Autodesk Fusion 360 part; units mm, degrees
sketch "Sketch1" plane through (0, 0, 0) normal (0, 0, 1) x (1, 0, 0)
sketch "Sketch2" plane through (0, 0, 0) normal (0, 0, 1) x (1, 0, 0)
  line L0 (-5, -5) -> (95, -5)
  line L1 (95, -5) -> (95, 13)
  line L2 (95, 13) -> (-5, 13)
  line L3 (-5, 13) -> (-5, -5)
  line L4 (-5, 13) -> (11, 13)
  line L5 (95, 13) -> (79, 13)
  line L6 (11, 13) -> (79, 13)
  line L7 (79, 13) -> (79, 19)
  line L8 (79, 19) -> (11, 19)
  line L9 (11, 19) -> (11, 13)
  line L10 (11, -5) -> (79, -5)
  line L11 (79, -5) -> (79, -11)
  line L12 (79, -11) -> (11, -11)
  line L13 (11, -11) -> (11, -5)
  line L14 (11, -11) -> (-5, -5)
  line L15 (-5, 13) -> (11, 19)
  line L16 (79, 19) -> (95, 13)
  line L17 (95, -5) -> (79, -11)
  dimension "d1" = 100
  dimension "d2" = 18
  dimension "d3" = 16
  dimension "d4" = 16
  dimension "d5" = 68
  dimension "d6" = 6
  dimension "d7" = 68
  dimension "d8" = 6
extrude "Extrude1" add sketch "Sketch2" along normal blind 20
sketch "Sketch3" plane through (95, 0, 0) normal (1, 0, 0) x (0, 1, 0)
  line L0 (-5, 0) -> (13, 0)
  line L1 (13, 0) -> (13, 20)
  line L2 (13, 20) -> (-5, 20)
  line L3 (-5, 20) -> (-5, 0)
  line L4 (-5, 20) -> (4, 20)
  arc A0 (-5, 20) -> (13, 20) centre (4, 20) ccw
  dimension "d11" = 9
  dimension "d12" = 18
extrude "Extrude2" cut sketch "Sketch3" against normal blind 100 contours L2 L4 A0
sketch "Sketch4" plane through (0, 0, 0) normal (0, 0, 1) x (1, 0, 0)
  line L0 (79, -11) -> (69.5, -11)
  line L1 (69.5, -11) -> (69.5, 19)
  line L2 (69.5, 19) -> (79, 19)
  line L3 (79, 19) -> (79, -11)
  line L4 (11, -11) -> (20.5, -11)
  line L5 (20.5, -11) -> (20.5, 19)
  line L6 (20.5, 19) -> (11, 19)
  line L7 (11, 19) -> (11, -11)
  line L8 (20.5, -11) -> (32.5, -11)
  line L9 (32.5, -11) -> (32.5, 19)
  line L10 (32.5, 19) -> (20.5, 19)
  line L11 (20.5, 19) -> (20.5, -11)
  line L12 (69.5, -11) -> (57.5, -11)
  line L13 (57.5, -11) -> (57.5, 19)
  line L14 (57.5, 19) -> (69.5, 19)
  line L15 (69.5, 19) -> (69.5, -11)
  dimension "d15" = 9.5
  dimension "d16" = 30
  dimension "d17" = 9.5
  dimension "d18" = 30
  dimension "d19" = 12
  dimension "d20" = 30
  dimension "d21" = 12
  dimension "d22" = 30
extrude "Extrude3" add sketch "Sketch4" against normal blind 25 contours L1 L12 L13 L14 L15 | L5 L8 L9 L10 L11
sketch "Sketch5" plane through (13.3562, -35.6164, 0) normal (0.3511, -0.9363, 0) x (0.9363, 0.3511, 0)
  line L0 (70.1076, 0) -> (87.1957, 0)
  line L1 (87.1957, 0) -> (87.1957, 20)
  line L2 (87.1957, 20) -> (70.1076, 20)
  line L3 (70.1076, 20) -> (70.1076, 0)
sketch "Sketch6" plane through (0, 0, 0) normal (0, 0, 1) x (1, 0, 0)
  line L0 (-5, -5) -> (95, -5)
  line L1 (95, -5) -> (95, -11)
  line L2 (95, -11) -> (-5, -11)
  line L3 (-5, -11) -> (-5, -5)
extrude "Extrude4" add sketch "Sketch6" along normal blind 20
Geometry check sheet. Reference: the model listing, model coordinates, mm. A direction names the side the tool comes from. Round coordinates to 2 decimals unless told otherwise and drop trailing zeros. Loops run counter-clockwise (first coordinate to the right, second up) from the corner with the lowest first, then second, coordinate; pieces in that order, holes last. Notation, with made-up numbers: (58, -35) - (75, -35) arc R28 ccw to (75, -11) - close; hole circle Ø5 at (-20.75, 60). An arc over 180 degrees is marked (long way). Write each question's results on one line, items separated by ' | '. Start each with the question number.
Q1. Access from +Z, -Z, +X, -X, +Y, -Y to the whole of each face (thin tool, end or side, straight path). Record for faces 1 (the flat face through (8, 4, 0)), 2 (the flat face through (32.5, 4, -12)), 3 (the flat face through (69.5, 4, -12)).
Q2. Cross-section at C-C on y = 4. Enter the section's corners in (x, z), and give its area (3 significant figures).
Q3. Gauge pin test, flat ends, axial feed: P1, Ø7.5, axis at y = 10.5, z = -14, coming from the +X side; P2, Ø7.5, axis at y = 10.5, z = -12, coming from the -X side; P3, Ø7.5, axis at x = 83, y = 3, coming from the -Z side. Record the tip position at first contact, or that the pin passes through.
Q4. Cross-section at D-D on z = 16. Enter the section's corners in (x, y).
Q5. Cross-section at A-A on z = -5. Enter the section's corners in (x, y).
Q6. Cross-section at B-B on x = 18. Enter the section's corners in (y, z).
Q7. Release check for a two-part mould opening along Y. For faces 4 (the cylindrical face through (46, 4, 11)), 5 (the flat face through (46, -11, 7)), 6 (the flat face through (-5, 1, 8)) record: +Y half, -Y half, draft (parallel to the pull), parting line (faces both ways), or undercut.
Q8. Thickness scan on line 1 (X direction, y = 11, z = -15); line 2 (Y direction, x = 61.5, z = 18); line 3 (Z direction, x = 53.5, y = -6). Record the ranges inside material, lowest first. Write a range as [from, to].
Answers below:
1) face 1: -Z, -X, +Y, -Y | face 2: -Z, +Y, -Y | face 3: -Z, +X, +Y, -Y
2) outline: (-5, 0) - (20.5, 0) - (20.5, -25) - (32.5, -25) - (32.5, 0) - (57.5, 0) - (57.5, -25) - (69.5, -25) - (69.5, 0) - (95, 0) - (95, 11) - (-5, 11) - close | area: 1,700 mm²
3) P1: stops at x = 69.5 | P2: stops at x = 20.5 | P3: stops at z = 0
4) outline: (-5, -11) - (95, -11) - (95, -4.06) - (-5, -4.06) - close; (-5, 12.06) - (95, 12.06) - (95, 13) - (79, 19) - (11, 19) - (-5, 13) - close
5) outline: (20.5, -11) - (32.5, -11) - (32.5, 19) - (20.5, 19) - close; (57.5, -11) - (69.5, -11) - (69.5, 19) - (57.5, 19) - close
6) outline: (-11, 0) - (19, 0) - (19, 20) - (13, 20) arc R9 cw to (-5, 20) - (-11, 20) - close
7) face 4: undercut | face 5: -Y half | face 6: draft
8) line 1: x = [20.5, 32.5], [57.5, 69.5] | line 2: y = [-11, -4.77], [12.77, 19] | line 3: z = [0, 20]
